Check sheet for the modelled part. Datum: model origin and axes. Units: mm. Face numbers are marked on the shaded views. A direction names the side the tool comes from. Round coordinates to 2 decimals unless told otherwise and drop trailing zeros. Loops run counter-clockwise (first coordinate to the right, second up) from the corner with the lowest first, then second, coordinate; pieces in that order, holes last. Notation, with made-up numbers: (80, -10) - (114, -10) arc R16 ccw to (114, 5) - close; hole circle Ø9 at (70.5, 60). An arc over 180 degrees is marked (long way). Put each result on its own line as item: value.
```python
from build123d import *

# Parameters (mm, degrees)
SKETCH1_R           = 2.5
BOSS_EXTRUDE1_DEPTH = 21
CUT_EXTRUDE2_DEPTH  = 4.5
SKETCH3_R           = 1
CUT_EXTRUDE3_DEPTH  = 6
CUT_EXTRUDE4_START  = -4.5
CUT_EXTRUDE4_DEPTH  = 4.5


with BuildPart() as part:
    # Sketch1 → Boss-Extrude1 (new body)
    with BuildSketch(Plane.XY):
        with Locations(Location((0, 0, 0), (0, 0, 180))):
            Circle(SKETCH1_R)
    extrude(amount=BOSS_EXTRUDE1_DEPTH)

    # Sketch2 → Cut-Extrude2 (cut)
    with BuildSketch(Plane(origin=(0, 0, 0), x_dir=(-1, 0, 0), z_dir=(0, 0, -1))):
        with BuildLine():
            Line((-1.75, -1.785357107), (-1.75, 1.785357107))
            ThreePointArc((-1.75, 1.785357107), (-2.5, 0), (-1.75, -1.785357107))
        make_face()
        with BuildLine():
            Line((1.75, -1.785357107), (1.75, 1.785357107))
            ThreePointArc((1.75, 1.785357107), (2.5, 0), (1.75, -1.785357107))
        make_face()
    extrude(amount=-CUT_EXTRUDE2_DEPTH, mode=Mode.SUBTRACT)

    # Sketch3 → Cut-Extrude3 (cut)
    with BuildSketch(Plane(origin=(0, 0, 0), x_dir=(-1, 0, 0), z_dir=(0, 0, -1))):
        Circle(SKETCH3_R)
    extrude(amount=-CUT_EXTRUDE3_DEPTH, mode=Mode.SUBTRACT)

    # Sketch4 → Cut-Extrude4 (cut)
    with BuildSketch(Plane.XY.offset(21).offset(CUT_EXTRUDE4_START)):
        with BuildLine():
            Line((-1.75, -1.785357107), (-1.75, 1.785357107))
            ThreePointArc((-1.75, 1.785357107), (-2.5, 0), (-1.75, -1.785357107))
        make_face()
    extrude(amount=CUT_EXTRUDE4_DEPTH, mode=Mode.SUBTRACT)


solid = part.part
```
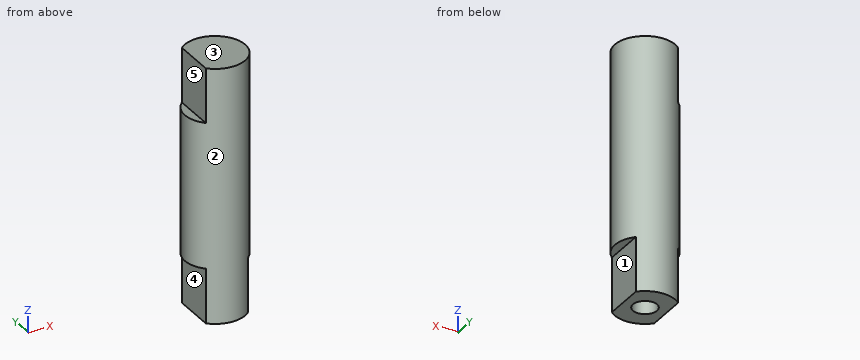
Item 1: Section check B-B on x = 0. Enter the section's corners in (y, z).
Filled sheet:
outline: (-2.5, 0) - (-1, 0) - (-1, 6) - (1, 6) - (1, 0) - (2.5, 0) - (2.5, 21) - (-2.5, 21) - close
Item 2: Go/stop test with flat-tipped pins: pin 1 (0.6 mm diameter, centred on x = 2, y = -0.5, fed in from -Z); pin 2 (1.1 mm diameter, centred on y = 0.5, z = 18.5, fed in from -X); pin 3 (1.8 mm diameter, centred on y = -0.5, z = 3, fed in from +X); pin 4 (0.8 mm diameter, centred on x = -2.5, y = 0, fed in from +Z). Record where each tip stops, or that it passes through.
Filled sheet:
pin 1: z = 0
pin 2: x = -1.75
pin 3: x = 1.75
pin 4: z = 16.5
Item 3: Section check A-A on y = -1.5. Enter the section's corners in (x, z), then the cut area to 3 significant figures.
Filled sheet:
outline: (-2, 4.5) - (-1.75, 4.5) - (-1.75, 0) - (1.75, 0) - (1.75, 4.5) - (2, 4.5) - (2, 21) - (-1.75, 21) - (-1.75, 16.5) - (-2, 16.5) - close
area: 80.6 mm²
Item 4: Thickness scan on line 1 (Y direction, x = 0, z = 2); line 2 (X direction, y = 0.1, z = 1); line 3 (Z direction, x = 0.1, y = 0.5). Record the ranges inside material, lowest first. Write a range as from..to.
Filled sheet:
line 1: -2.5..-1, 1..2.5
line 2: -1.75..-0.99, 0.99..1.75
line 3: 6..21
Item 5: Section check C-C on z = 5.5. Enter the section's corners in (x, y), then the cut area to 3 significant figures.
Filled sheet:
outline: circle Ø5 at (0, 0); hole circle Ø2 at (0, 0)
area: 16.5 mm²
Item 6: Section check D-D on y = 0. Enter the section's corners in (x, z), then the cut area to 3 significant figures.
Filled sheet:
outline: (-2.5, 4.5) - (-1.75, 4.5) - (-1.75, 0) - (-1, 0) - (-1, 6) - (1, 6) - (1, 0) - (1.75, 0) - (1.75, 4.5) - (2.5, 4.5) - (2.5, 21) - (-1.75, 21) - (-1.75, 16.5) - (-2.5, 16.5) - close
area: 82.9 mm²
Item 7: Tool access check on the marked faces 1, 2, 3, 4 and 5. Record the directions out of +Z, -Z, +X, -X, +Y, -Y that give a thin tool (end or side, any length) a straight path to the whole face; none if there is none.
Filled sheet:
face 1: -Z, +X, +Y, -Y
face 2: +Z, -Z
face 3: +Z, +X, -X, +Y, -Y
face 4: -Z, -X, +Y, -Y
face 5: +Z, -X, +Y, -Y
